```python
from build123d import *

# Parameters (mm, degrees)
SKETCH_1_R          = 33
EXTRUDE_1_DEPTH     = 20
CUT_EXTRUDE_2_DEPTH = 25
SKETCH_1_6_R        = 21
CUT_EXTRUDE_3_DEPTH = 16
CUT_EXTRUDE_5_DEPTH = 30


with BuildPart() as part:
    # 草图1 → 凸台-拉伸1 (new body)
    with BuildSketch(Plane.XY):
        Circle(SKETCH_1_R)
    extrude(amount=EXTRUDE_1_DEPTH)

    # 草图1<5> → 切除-拉伸2 (cut, symmetric)
    with BuildSketch(Plane.XY):
        with BuildLine():
            ThreePointArc((-8, -8.94427191), (-8.929533731, -8.377822811), (-10, -8.180339887))
            ThreePointArc((-10, -8.180339887), (-12.802517077, -10.109873618), (-12, -13.416407865))
            ThreePointArc((-12, -13.416407865), (0, -18), (12, -13.416407865))
            ThreePointArc((12, -13.416407865), (12.802517077, -10.109873618), (10, -8.180339887))
            ThreePointArc((10, -8.180339887), (8.929533731, -8.377822811), (8, -8.94427191))
            ThreePointArc((8, -8.94427191), (0, -12), (-8, -8.94427191))
        make_face()
        with BuildLine():
            ThreePointArc((-12, 13.416407865), (-12.236067977, 9.180339887), (-8, 8.94427191))
            ThreePointArc((-8, 8.94427191), (-4.281865077, 11.210068308), (0, 12))
            ThreePointArc((0, 12), (4.281865077, 11.210068308), (8, 8.94427191))
            ThreePointArc((8, 8.94427191), (12.236067977, 9.180339887), (12, 13.416407865))
            ThreePointArc((12, 13.416407865), (6.422797616, 16.815102461), (0, 18))
            ThreePointArc((0, 18), (-6.422797616, 16.815102461), (-12, 13.416407865))
        make_face()
    extrude(amount=CUT_EXTRUDE_2_DEPTH, both=True, mode=Mode.SUBTRACT)

    # 草图1<6> → 切除-拉伸3 (cut)
    with BuildSketch(Plane.XY):
        Circle(SKETCH_1_6_R)
    extrude(amount=CUT_EXTRUDE_3_DEPTH, mode=Mode.SUBTRACT)

    # 草图1<7> → 切除-拉伸5 (cut, symmetric)
    with BuildSketch(Plane.XY):
        with BuildLine():
            ThreePointArc((0, 8.05), (-1.55, 6.5), (0, 4.95))
            ThreePointArc((0, 4.95), (1.55, 6.5), (0, 8.05))
        make_face()
        with BuildLine():
            ThreePointArc((0, -4.95), (-1.55, -6.5), (0, -8.05))
            ThreePointArc((0, -8.05), (1.55, -6.5), (0, -4.95))
        make_face()
        with BuildLine():
            ThreePointArc((6, 1.55), (4.45, 0), (6, -1.55))
            ThreePointArc((6, -1.55), (7.55, 0), (6, 1.55))
        make_face()
        with BuildLine():
            ThreePointArc((-6, 1.55), (-7.55, 0), (-6, -1.55))
            ThreePointArc((-6, -1.55), (-4.45, 0), (-6, 1.55))
        make_face()
        with BuildLine():
            ThreePointArc((0, 4.15), (-4.15, 0), (0, -4.15))
            ThreePointArc((0, -4.15), (4.15, 0), (0, 4.15))
        make_face()
    extrude(amount=CUT_EXTRUDE_5_DEPTH, both=True, mode=Mode.SUBTRACT)


solid = part.part
```
Geometry check sheet. Reference: the model listing, model coordinates, mm. A direction names the side the tool comes from. Give positions to 0.01 mm unless a question says otherwise; leave off trailing zeros. Write each loop counter-clockwise with the first axis right and the second up, starting at its lowest first coordinate (ties: lowest second). Pieces come first, ordered by that corner, then holes. Notation, with made-up numbers: (7, 40.5) - (33, 40.5) arc R26 cw to (33, 76.5) - close; hole circle Ø10 at (33, -36.5). An arc over 180 degrees is marked (long way). Use a Markdown table: item, result.
Q1. Section check A-A, the plane y = 0. Enter the section's corners in (x, z), then the cut area to 3 significant figures.
Computed:
| item | result |
|---|---|
| outline | (-33, 0) - (-21, 0) - (-21, 16) - (-7.55, 16) - (-7.55, 20) - (-33, 20) - close; (-4.45, 16) - (-4.15, 16) - (-4.15, 20) - (-4.45, 20) - close; (4.15, 16) - (4.45, 16) - (4.45, 20) - (4.15, 20) - close; (7.55, 16) - (21, 16) - (21, 0) - (33, 0) - (33, 20) - (7.55, 20) - close |
| area | 590 mm² |
Q2. Section check B-B, the plane z = 17.25. Enter the section's corners in (x, y), then the cut area to 3 significant figures.
Computed:
| item | result |
|---|---|
| outline | circle Ø66 at (0, 0); hole (-12, -13.42) arc R18 ccw to (12, -13.42) arc R3 ccw to (8, -8.94) arc R12 cw to (-8, -8.94) arc R3 ccw to start; hole (-12, 13.42) arc R3 ccw to (-8, 8.94) arc R12 cw to (8, 8.94) arc R3 ccw to (12, 13.42) arc R18 ccw to start; hole circle Ø3.1 at (-6, 0); hole circle Ø8.3 at (0, 0); hole circle Ø3.1 at (0, -6.5); hole circle Ø3.1 at (0, 6.5); hole circle Ø3.1 at (6, 0) |
| area | 3,020 mm² |
Q3. Go/stop test with flat-tipped pins: P1, Ø5, axis at y = 11.5, z = 5.5, coming from the -X side; P2, Ø1.5, axis at x = 24.5, z = 13, coming from the +Y side; P3, Ø12, axis at y = -14.5, z = 12, coming from the +X side. Record where each tip stops, or that it passes through.
Computed:
| item | result |
|---|---|
| P1 | stops at x = -31.75 |
| P2 | stops at y = 22.91 |
| P3 | stops at x = 31.89 |
Q4. Thickness scan on L1, parallel to Y at x = 0, z = 10.25; L2, parallel to Z at x = 3, y = 20.5; L3, parallel to Y at x = 8, z = 8. Record the ranges inside material, lowest first. Write a range as [from, to].
Computed:
| item | result |
|---|---|
| L1 | y = [-33, -21], [21, 33] |
| L2 | z = [16, 20] |
| L3 | y = [-32.02, -19.42], [19.42, 32.02] |
Q5. Section check C-C, the plane x = -2.5. Enter the section's corners in (y, z).
Computed:
| item | result |
|---|---|
| outline | (-32.91, 0) - (-20.85, 0) - (-20.85, 16) - (-17.83, 16) - (-17.83, 20) - (-32.91, 20) - close; (-11.74, 16) - (-3.31, 16) - (-3.31, 20) - (-11.74, 20) - close; (3.31, 16) - (11.74, 16) - (11.74, 20) - (3.31, 20) - close; (17.83, 16) - (20.85, 16) - (20.85, 0) - (32.91, 0) - (32.91, 20) - (17.83, 20) - close |
Q6. Section check D-D, the plane z = 1.5. Enter the section's corners in (x, y).
Computed:
| item | result |
|---|---|
| outline | circle Ø66 at (0, 0); hole circle Ø42 at (0, 0) |
Q7. Set-up check for faces 5 (the face through (0, -18, 18)), 6 (the face through (20.03, 6.31, 7.89)), 7 (the face through (-8, 0, 20)): record each of +Z, -Z, +X, -X, +Y, -Y from which the full face is reachable in a straight line by a thin tool's end or side.
Computed:
| item | result |
|---|---|
| face 5 | +Z, -Z |
| face 6 | -Z |
| face 7 | +Z, +X, -X, +Y, -Y |
Q8. Draft check along X on faces 1 (the face through (30.5, -12.6, 9.9)), 2 (the face through (0, -22, 0)), 3 (the face through (0.07, -4.95, 17.97)), 4 (the face through (-12.28, 9.23, 18.03)). Enter one of: pulls with the +X half, pulls with the -X half, needs draft (parallel to the pull), parting line crosses it, or undercut.
Computed:
| item | result |
|---|---|
| face 1 | parting line crosses it |
| face 2 | needs draft |
| face 3 | undercut |
| face 4 | undercut |
